For this review, take the finished solid that the model builds, in its own axes (mm). Face numbers are marked on the shaded views. A direction names the side the tool comes from. Coordinates: 2 decimals unless noted, no trailing zeros. Loops run counter-clockwise (first coordinate to the right, second up) from the corner with the lowest first, then second, coordinate; pieces in that order, holes last. Notation, with made-up numbers: (13.5, -25) -> (58.5, -25) arc R30 ccw to (58.5, 10) -> close; hole circle Ø4 at (2, -17). An arc over 180 degrees is marked (long way). Answer in a Markdown table with one row per item.
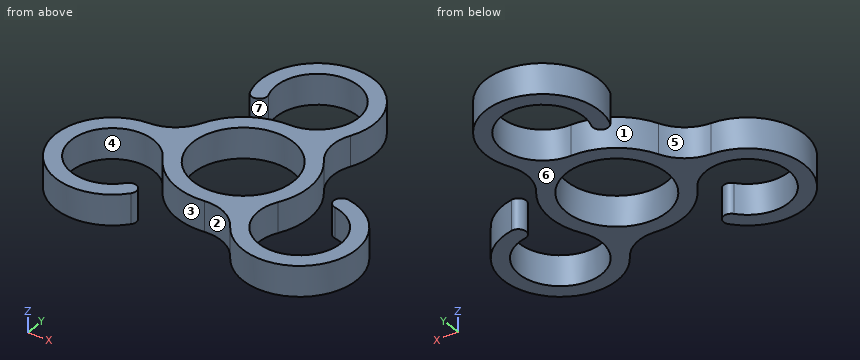
from build123d import *

# Parameters (mm, degrees)
F0_R     = 8
F1_DEPTH = 4.83


with BuildPart() as f1:
    # F0 (on Top) → F1 (new body)
    with BuildSketch(Plane.XY):
        with BuildLine():
            ThreePointArc((-6.154987, 14.809768), (3.756926, 22.415446), (0, 10.5))
            ThreePointArc((0, 10.5), (-5.692087, 8.823273), (-9.566255, 4.328598))
            ThreePointArc((-9.566255, 4.328598), (-11.838577, 1.629537), (-15.186217, 0.515226))
            ThreePointArc((-15.186217, 0.515226), (-22.876728, -12.539258), (-7.833031, -14.342228))
            ThreePointArc((-7.833031, -14.342228), (-7.987102, -12.581188), (-9.748142, -12.735259))
            ThreePointArc((-9.748142, -12.735259), (-21.290808, -7.95413), (-9.093267, -5.25))
            ThreePointArc((-9.093267, -5.25), (-4.795135, -9.341129), (1.034452, -10.448919))
            ThreePointArc((1.034452, -10.448919), (4.508068, -11.067277), (7.14691, -13.409263))
            ThreePointArc((7.14691, -13.409263), (22.29768, -13.542198), (16.337249, 0.38751))
            ThreePointArc((16.337249, 0.38751), (14.889179, -0.626439), (15.903129, -2.074509))
            ThreePointArc((15.903129, -2.074509), (17.533883, -14.461316), (9.093267, -5.25))
            ThreePointArc((9.093267, -5.25), (10.487222, 0.517856), (8.531804, 6.120321))
            ThreePointArc((8.531804, 6.120321), (7.330509, 9.43774), (8.039308, 12.894037))
            ThreePointArc((8.039308, 12.894037), (0.579048, 26.081456), (-8.504218, 13.954718))
            ThreePointArc((-8.504218, 13.954718), (-6.902077, 13.207627), (-6.154987, 14.809768))
        make_face()
        Circle(F0_R, mode=Mode.SUBTRACT)
    extrude(amount=F1_DEPTH)


solid = f1.part
Item 1: For L1, parallel to Y at x = 2, z = 1.6; L2, parallel to Y at x = -1, z = 1.2; L3, parallel to X at y = 17.05, z = 1.3, list the stretches that pass through material, from the lowest coordinate up.
Worked answers:
| item | result |
|---|---|
| L1 | -10.43 to -7.75, 7.75 to 10.81, 23.29 to 25.88 |
| L2 | -10.45 to -7.94, 7.94 to 10.45, 23.52 to 26.04 |
| L3 | -9.05 to -6.55, 6.55 to 9.05 |
Item 2: Take a section at D-D, the plane y = -3. State the section outline as (x, z) points, and give its area (3 significant figures).
Worked answers:
| item | result |
|---|---|
| outline | (-21.93, 0) -> (-18.28, 0) -> (-18.28, 4.83) -> (-21.93, 4.83) -> close; (-11.25, 0) -> (-7.42, 0) -> (-7.42, 4.83) -> (-11.25, 4.83) -> close; (7.42, 0) -> (10.06, 0) -> (10.06, 4.83) -> (7.42, 4.83) -> close; (18.28, 0) -> (21.93, 0) -> (21.93, 4.83) -> (18.28, 4.83) -> close |
| area | 66.5 mm² |
Item 3: The part is to be moulded in two halves that separate along X. For the marked faces 4, 5, 6 and 7, say which applies: +X half, -X half, draft (parallel to the pull), parting line (faces both ways), or undercut.
Worked answers:
| item | result |
|---|---|
| face 4 | undercut |
| face 5 | -X half |
| face 6 | draft |
| face 7 | undercut |
Item 4: Insertion check: pin 1 (2 mm diameter, centred on y = -2, z = 3, fed in from +X); pin 2 (2 mm diameter, centred on x = -18.5, y = 2, fed in from -Z); pin 3 (1.5 mm diameter, centred on x = 7.5, z = 1.5, fed in from -Y). Each pin has a flat end and moves straight along its axis. Give the tip position at first contact, or say it passes through.
Worked answers:
| item | result |
|---|---|
| pin 1 | x = 21.93 |
| pin 2 | through |
| pin 3 | y = -14.81 |
Item 5: For the marked faces 1, 2 and 3, list the 3-axis set-ups (+Z, -Z, +X, -X, +Y, -Y) from which the entire face can be reached by the end or side of a thin tool; tool diameter is ignored.
Worked answers:
| item | result |
|---|---|
| face 1 | +Z, -Z, -X |
| face 2 | +Z, -Z, -Y |
| face 3 | +Z, -Z |
Item 6: Take a section at A-A, the plane y = 17.05. State the section outline as (x, z) points.
Worked answers:
| item | result |
|---|---|
| outline | (-9.05, 0) -> (-6.55, 0) -> (-6.55, 4.83) -> (-9.05, 4.83) -> close; (6.55, 0) -> (9.05, 0) -> (9.05, 4.83) -> (6.55, 4.83) -> close |
Item 7: Take a section at B-B, the plane x = -11. State the section outline as (y, z) points.
Worked answers:
| item | result |
|---|---|
| outline | (-16.75, 0) -> (-13.88, 0) -> (-13.88, 4.83) -> (-16.75, 4.83) -> close; (-3.17, 0) -> (2.31, 0) -> (2.31, 4.83) -> (-3.17, 4.83) -> close |
